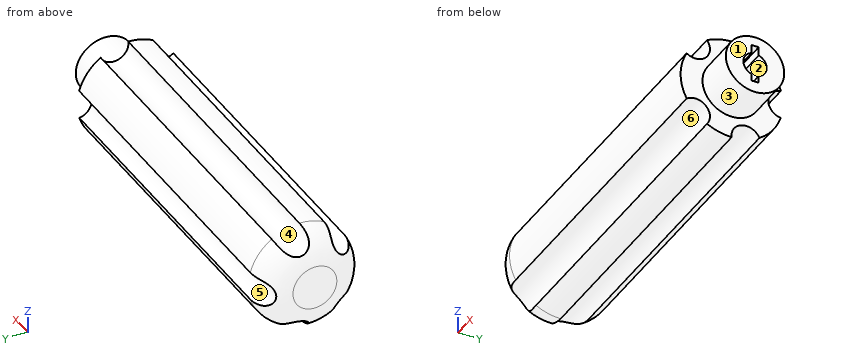
Solid Edge part; units mm, degrees
sketch "Sketch1" plane through (0, 0, 0) normal (1, 0, 0) x (0, 1, 0)
  circle A0 centre (0, 0) radius 10
extrude "Protrusion1" add sketch "Sketch1" along normal blind 15
sketch "Sketch2" plane through (0, 0, 0) normal (1, 0, 0) x (0, 1, 0)
  circle A0 centre (0, 0) radius 17.5
extrude "拉伸_6" add sketch "Sketch2" against normal blind 120
fillet "倒圆_1" radius 10 1 edges at (-120, -17.5, 0)
sketch "Sketch3" plane through (0, 0, 0) normal (1, 0, 0) x (0, 0, 1)
  circle A0 centre (-0.1208, -17.4996) radius 5
  circle A1 centre (16.7876, -4.9424) radius 5
  circle A2 centre (-16.7876, -4.9424) radius 5
  circle A3 centre (12.3049, 12.4434) radius 5
  circle A4 centre (-12.3049, 12.4434) radius 5
extrude "Cutout1" cut sketch "Sketch3" against normal up to vertex (120 mm away)
sketch "Sketch4" plane through (0, 0, 0) normal (1, 0, 0) x (0, 1, 0)
  circle A0 centre (0, 0) radius 4
  line L0 (-1.2419, -6.2095) -> (1.2581, -6.2095)
  line L1 (1.2581, -6.2095) -> (1.2581, 6.7905)
  line L2 (1.2581, 6.7905) -> (-1.2419, 6.7905)
  line L3 (-1.2419, 6.7905) -> (-1.2419, -6.2095)
extrude "拉伸除料_3" cut sketch "Sketch4" along normal blind 15
properties material "ABS 高抗冲击塑料"
Source: CAD feature listing. Evaluate the final solid. Frame: model axes, mm. Face numbers are marked on the shaded views. A direction names the side the tool comes from. Give positions to 0.01 mm unless a question says otherwise; leave off trailing zeros. Loops run counter-clockwise (first coordinate to the right, second up) from the corner with the lowest first, then second, coordinate; pieces in that order, holes last. Notation, with made-up numbers: (72.5, 77) -> (115.5, 77) arc R19 ccw to (115.5, 81) -> close; hole circle Ø2 at (80, 87.5). An arc over 180 degrees is marked (long way). Use a Markdown table: item, result. Add a question column.
(1) First-contact query: pin 1 Ø1.5 at (x, z) = (8.5, 5) entering from -Y; pin 2 Ø5 at (x, y) = (-1, -6.5) entering from -Z; pin 3 Ø0.7 at (x, z) = (6, -5.5) entering from -Y; pin 4 Ø12 at (x, y) = (-80.5, -0.5) entering from +Z. Flat tips, straight axial feed; report the tip coordinate or a pass-through.
(2) Access query for the marked faces 1 and 2. Directions: +Z, -Z, +X, -X, +Y, -Y. A direction counts if a zero-diameter tool reaches every point of the face in a straight line with its end or side. Return the directions, or none.
(3) Pull-direction query (Y, two-part tool) for the marked faces 3, 4, 5 and 6; classes: +Y half, -Y half, draft (parallel to the pull), parting line (faces both ways), or undercut.
(4) Ray query, line 1 (Z direction, x = -84, y = -8); line 2 (X direction, y = -2, z = -1); line 3 (Z direction, x = -82, y = 14). Return the intervals inside material, ascending.
(5) Section query A-A (x = -84). Output: boundary loops of the cut face in (y, z).
Checked values:
| question | item | result |
|---|---|---|
| 1 | pin 1 | y = -9.05 |
| 1 | pin 2 | z = -17.04 |
| 1 | pin 3 | y = -8.57 |
| 1 | pin 4 | z = 17.5 |
| 2 | face 1 | +Z, -Z, +X, +Y, -Y |
| 2 | face 2 | +X |
| 3 | face 3 | parting line |
| 3 | face 4 | undercut |
| 3 | face 5 | +Y half |
| 3 | face 6 | undercut |
| 4 | line 1 | -15.56 to -14.6, -10.01 to 10.01, 14.6 to 15.56 |
| 4 | line 2 | -120 to 0 |
| 4 | line 3 | -10.5 to -3.69, 3.45 to 10.5 |
| 5 | outline | (-15.42, -8.28) arc R5 cw to (-8.46, -15.32) arc R17.5 ccw to (-0.01, -17.5) arc R5 cw to (9.49, -14.7) arc R17.5 ccw to (16.75, -5.06) arc R5 cw to (16.82, 4.83) arc R17.5 ccw to (9.49, 14.7) arc R5 cw to (-0.01, 17.5) arc R17.5 ccw to (-8.46, 15.32) arc R5 cw to (-15.42, 8.28) arc R17.5 ccw to start |
